Model file for the job. Use its own axes, mm. Coordinates: 2 decimals unless noted, no trailing zeros. Write each loop counter-clockwise with the first axis right and the second up, starting at its lowest first coordinate (ties: lowest second). Pieces come first, ordered by that corner, then holes.
Q1. Pin check, flat tips, straight feed: P1, Ø1.5, axis at x = 52.5, z = 2, coming from the -Y side; P2, Ø3, axis at y = -28, z = 3.5, coming from the -X side; P3, Ø2, axis at x = 2, z = 1.5, coming from the -Y side. Stop position of each tip, or through.
Q2. Band-saw the part on A-A, the plane z = 1.95. Write the cut outline in (x, y).
Q3. Drill centre lines: probe 1 along X at (y, z) = (5.5, 1.6); probe 2 along X at (y, z) = (4, 2.9); probe 3 along X at (y, z) = (2, 4.2). Where is each one in solid material? Low to high.
Q4. Band-saw the part on B-B, the plane y = -23. Write the cut outline in (x, z).
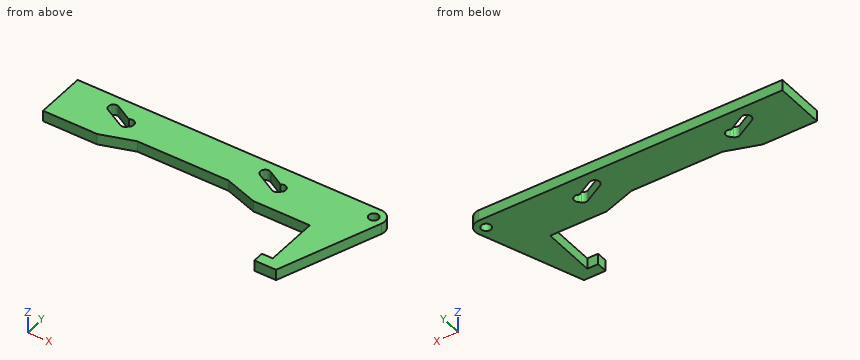
from build123d import *

# Parameters (mm, degrees)
SKETCH1_W           = 16
SKETCH1_H           = 5
BOSS_EXTRUDE1_DEPTH = 5
SKETCH2_W           = 42
SKETCH2_H           = 5
CUT_EXTRUDE1_DEPTH  = 5
SKETCH3_R           = 5
SKETCH3_R_2         = 2.25
BOSS_EXTRUDE2_DEPTH = 5


with BuildPart() as part:
    # Sketch1 → Boss-Extrude1 (new body)
    with BuildSketch(Plane.XY):
        with BuildLine():
            Line((-41.677050983, 9), (-45, 9))
            Line((-45, 9), (-61, 9))
            Line((-61, 9), (-61, -9))
            Line((-61, -9), (61, -9))
            Line((61, -9), (61, 9))
            Line((61, 9), (45, 9))
            Line((45, 9), (31.933033563, 9))
            Line((31.933033563, 9), (38.62595316, 5.281711335))
            ThreePointArc((38.62595316, 5.281711335), (40.992696986, 5.519171289), (42.25, 3.5))
            ThreePointArc((42.25, 3.5), (42.078728948, 2.638962277), (41.590990258, 1.909009742))
            Line((41.590990258, 1.909009742), (40.590990258, 0.909009742))
            ThreePointArc((40.590990258, 0.909009742), (39.312077727, 0.271747884), (37.907303405, 0.533146129))
            Line((37.907303405, 0.533146129), (28.907303405, 5.533146129))
            ThreePointArc((28.907303405, 5.533146129), (27.781296696, 7.126027211), (28.322949017, 9))
            Line((28.322949017, 9), (-38.066966437, 9))
            Line((-38.066966437, 9), (-31.37404684, 5.281711335))
            ThreePointArc((-31.37404684, 5.281711335), (-29.007303014, 5.519171289), (-27.75, 3.5))
            ThreePointArc((-27.75, 3.5), (-27.921271052, 2.638962277), (-28.409009742, 1.909009742))
            Line((-28.409009742, 1.909009742), (-29.409009742, 0.909009742))
            ThreePointArc((-29.409009742, 0.909009742), (-30.687922273, 0.271747884), (-32.092696595, 0.533146129))
            Line((-32.092696595, 0.533146129), (-41.092696595, 5.533146129))
            ThreePointArc((-41.092696595, 5.533146129), (-42.218703304, 7.126027211), (-41.677050983, 9))
        make_face()
        with BuildLine():
            Line((45, 14), (-45, 14))
            Line((-45, 14), (-45, 9))
            Line((-45, 9), (-41.677050983, 9))
            ThreePointArc((-41.677050983, 9), (-40.373972789, 9.718703304), (-38.907303405, 9.466853871))
            Line((-38.907303405, 9.466853871), (-38.066966437, 9))
            Line((-38.066966437, 9), (28.322949017, 9))
            ThreePointArc((28.322949017, 9), (29.626027211, 9.718703304), (31.092696595, 9.466853871))
            Line((31.092696595, 9.466853871), (31.933033563, 9))
            Line((31.933033563, 9), (45, 9))
            Line((45, 9), (45, 14))
        make_face()
        with Locations((-53, 11.5)):
            Rectangle(SKETCH1_W, SKETCH1_H)
        with Locations((53, 11.5)):
            Rectangle(SKETCH1_W, SKETCH1_H)
    extrude(amount=BOSS_EXTRUDE1_DEPTH)

    # Sketch2 → Cut-Extrude1 (cut)
    with BuildSketch(Plane.XY.offset(5)):
        Polygon((-36, -9), (-21, -9), (-21, -4), align=None)
        with Locations((0, -6.5)):
            Rectangle(SKETCH2_W, SKETCH2_H)
        Polygon((21, -4), (21, -9), (36, -9), align=None)
    extrude(amount=-CUT_EXTRUDE1_DEPTH, mode=Mode.SUBTRACT)

    # Sketch3 → Boss-Extrude2 (add)
    # profile 1 of 2: a face of its own
    with BuildSketch(Plane.XY.offset(5)):
        with Locations((79, 9)):
            Circle(SKETCH3_R)
        with Locations((79, 9)):
            Circle(SKETCH3_R_2, mode=Mode.SUBTRACT)
    # profile 2 of 2: a face of its own
    with BuildSketch(Plane.XY.offset(5)):
        with BuildLine():
            Line((79, 14), (61, 14))
            Line((61, 14), (61, -9))
            Line((61, -9), (62, -9))
            Line((62, -9), (62, -33.65))
            Line((62, -33.65), (57, -33.65))
            Line((57, -33.65), (57, -38.65))
            Line((57, -38.65), (67, -38.65))
            Line((67, -38.65), (83.699195541, 7.29191298))
            ThreePointArc((83.699195541, 7.29191298), (74.904854392, 6.131240259), (79, 14))
        make_face()
    extrude(amount=-BOSS_EXTRUDE2_DEPTH)


solid = part.part
Answer sheet:
1. P1: stops at y = -9
1. P2: stops at x = 62
1. P3: stops at y = -4
2. outline: (-61, -9) - (-36, -9) - (-21, -4) - (21, -4) - (36, -9) - (62, -9) - (62, -33.65) - (57, -33.65) - (57, -38.65) - (67, -38.65) - (83.7, 7.29) arc R5 ccw to (79, 14) - (-61, 14) - close; hole (-41.09, 5.53) - (-32.09, 0.53) arc R2.25 ccw to (-29.41, 0.91) - (-28.41, 1.91) arc R2.25 ccw to (-31.37, 5.28) - (-38.91, 9.47) arc R2.25 ccw to start; hole (28.91, 5.53) - (37.91, 0.53) arc R2.25 ccw to (40.59, 0.91) - (41.59, 1.91) arc R2.25 ccw to (38.63, 5.28) - (31.09, 9.47) arc R2.25 ccw to start; hole circle Ø4.5 at (79, 9)
3. probe 1: x = -61 to -41.03, -31.77 to -31.03, -28.97 to 28.97, 38.23 to 38.97, 41.03 to 83.05
3. probe 2: x = -61 to -38.33, -27.81 to 31.67, 42.19 to 82.5
3. probe 3: x = -61 to -34.73, -28.32 to 35.27, 41.68 to 81.78
4. outline: (62, 0) - (72.69, 0) - (72.69, 5) - (62, 5) - close
